Verification items for the finished model (mm, model axes). A direction names the side the tool comes from. Coordinates: 2 decimals unless noted, no trailing zeros. Order: outer loops, then holes, each group sorted by start corner. A loop starts at its lowest first (then second) coordinate and runs counter-clockwise, first axis right, second up. Notation, with made-up numbers: (-29.5, 71.5) - (-6.5, 71.5) arc R11 cw to (-6.5, 86.5) - close; hole circle Ø8 at (-15.75, 44.5). An arc over 180 degrees is marked (long way). Answer as CSV lines item,"result". Start each with the question number.
1. Set-up check for faces 5 (the flat face through (-100, -26, -142)), 6 (the flat face through (7.3, -15.1, -605)), 7 (the cylindrical face through (-15.738, -4.956, 3.479)), 8 (the flat face through (-100, -3, 18)), 9 (the cylindrical face through (124.307, -4.506, -623.07)): record each of +Z, -Z, +X, -X, +Y, -Y from which the full face is reachable in a straight line by a thin tool's end or side.
2. Section check A-A (z = -550). Record the cut outline in (x, y), and give its area (3 significant figures).
3. Material ranges on L1, parallel to Y at x = 0, z = -602.65; L2, parallel to Y at x = 0, z = -601; L3, parallel to X at y = 6.5, z = -95.5, recorded low to high. Write a range as [from, to].
4. Section check B-B (y = -63). Record the cut outline in (x, z).
5. Go/stop test with flat-tipped pins: pin 1 (5 mm diameter, centred on x = 73, z = -541.5, fed in from +Y); pin 2 (3.5 mm diameter, centred on x = 0, y = -25, fed in from +Z); pin 3 (2 mm diameter, centred on x = -24, y = -1, fed in from -Z). Record where each tip stops, or that it passes through.
6. Section check D-D (x = 110). Record the cut outline in (y, z).
7. Mould release check, pull along Z, two halves, no side actions. Record for faces 1 (the cylindrical face through (-95.693, 4.506, 22.93)), 2 (the cylindrical face through (120, 0, -609)), 3 (the cylindrical face through (-4.56, -34.7, -550.38)), 4 (the flat face through (0, 0, 2)): pulls with the +Z half, pulls with the -Z half, needs draft (parallel to the pull), parting line crosses it, or undercut.
from build123d import *

# Parameters (mm, degrees)
SKETCH3_W            = 300
SKETCH3_H            = 200
BOSS_EXTRUDE2_DEPTH  = 300
SKETCH8_R            = 35
SKETCH8_R_2          = 2
SKETCH8_R_3          = 2.3
BOSS_EXTRUDE7_DEPTH  = 5
BOSS_EXTRUDE8_DEPTH  = 300
SKETCH19_W           = 200
SKETCH19_H           = 260
CUT_EXTRUDE5_DEPTH   = 150
CUT_EXTRUDE3_REACH   = 673.584
CUT_EXTRUDE4_DEPTH   = 200
CHAMFER2_SIZE        = 50
SKETCH4_R            = 10
BOSS_EXTRUDE9_DEPTH  = 18
SKETCH15_R           = 15
BOSS_EXTRUDE10_DEPTH = 10
BOSS_EXTRUDE11_START = 18
SKETCH16_R           = 10
BOSS_EXTRUDE11_DEPTH = 18
BOSS_EXTRUDE12_START = 10
SKETCH17_R           = 15
BOSS_EXTRUDE12_DEPTH = 10
SKETCH18_R           = 75
BOSS_EXTRUDE13_DEPTH = 10
CUT_EXTRUDE6_REACH   = 685.318
SKETCH20_R           = 35
SKETCH21_R           = 16.5
CUT_EXTRUDE7_DEPTH   = 3
CUT_EXTRUDE8_START   = -3
SKETCH22_R           = 16.5
CUT_EXTRUDE8_DEPTH   = 3
SKETCH23_R           = 2
SKETCH23_R_2         = 2.3
CUT_EXTRUDE9_DEPTH   = 20


with BuildPart() as part:
    # Sketch3 → Boss-Extrude2 (new body)
    with BuildSketch(Plane.XY):
        Rectangle(SKETCH3_W, SKETCH3_H)
    extrude(amount=-BOSS_EXTRUDE2_DEPTH)

    # Sketch8 → Boss-Extrude7 (add)
    with BuildSketch(Plane.XY):
        Circle(SKETCH8_R)
        with Locations((0, 25)):
            Circle(SKETCH8_R_2, mode=Mode.SUBTRACT)
        with Locations((0, -25)):
            Circle(SKETCH8_R_2, mode=Mode.SUBTRACT)
        with Locations((25, 0)):
            Circle(SKETCH8_R_3, mode=Mode.SUBTRACT)
        with Locations((-25, 0)):
            Circle(SKETCH8_R_2, mode=Mode.SUBTRACT)
    extrude(amount=BOSS_EXTRUDE7_DEPTH)

    # Mirror1: part across plane


with BuildPart() as part_1:
    add(part.part)
    add(part.part.mirror(Plane(origin=(0, 0, -300), x_dir=(1, 0, 0), z_dir=(0, 0, -1))))

    # Sketch10 → Boss-Extrude8 (add)
    with BuildSketch(Plane(origin=(150, 0, 0), x_dir=(0, 0, -1), z_dir=(1, 0, 0))):
        Polygon((0, 100), (400, 250), (600, 100), align=None)
    extrude(amount=-BOSS_EXTRUDE8_DEPTH)

    # Sketch19 → Cut-Extrude5 (cut)
    with BuildSketch(Plane.XZ.offset(100)):
        with Locations((0, -140)):
            Rectangle(SKETCH19_W, SKETCH19_H)
    extrude(amount=-CUT_EXTRUDE5_DEPTH, mode=Mode.SUBTRACT)

    # Cut-Extrude3: up to this plane
    cut_extrude3_end = Plane(origin=(-768.465843843, 250, -400), z_dir=(0, 0.7999999999999999, -0.6000000000000001))
    # Sketch11 → Cut-Extrude3 (cut, up to the surface)
    with BuildSketch(Plane.XY, mode=Mode.PRIVATE) as cut_extrude3_sk1:
        Polygon((150, 100), (95.40446486, 250), (150, 250), align=None)
    cut_extrude3_tool1 = split(extrude(cut_extrude3_sk1.sketch, amount=-CUT_EXTRUDE3_REACH, mode=Mode.PRIVATE), bisect_by=cut_extrude3_end, keep=Keep.BOTH, mode=Mode.PRIVATE)
    add(cut_extrude3_tool1.solids().sort_by_distance((131.801488, 200, 0))[0], mode=Mode.SUBTRACT)
    # Sketch11 → Cut-Extrude3 (cut, up to the surface)
    with BuildSketch(Plane.XY, mode=Mode.PRIVATE) as cut_extrude3_sk2:
        Polygon((-150, 100), (-95.40446486, 250), (-150, 250), align=None)
    cut_extrude3_tool2 = split(extrude(cut_extrude3_sk2.sketch, amount=-CUT_EXTRUDE3_REACH, mode=Mode.PRIVATE), bisect_by=cut_extrude3_end, keep=Keep.BOTH, mode=Mode.PRIVATE)
    add(cut_extrude3_tool2.solids().sort_by_distance((-131.801488, 200, 0))[0], mode=Mode.SUBTRACT)

    # Sketch14 → Cut-Extrude4 (cut)
    with BuildSketch(Plane(origin=(0, 352, -264), x_dir=(1, 0, 0), z_dir=(0, 0.7999999999999999, -0.6000000000000002))):
        Polygon((-137.580501971, 410), (137.580501971, 410), (87.352609643, 180), (-87.352609643, 180), align=None)
    extrude(amount=-CUT_EXTRUDE4_DEPTH, mode=Mode.SUBTRACT)

    # Chamfer2
    chamfer2_edges = [part_1.edges().sort_by_distance(p)[0] for p in [
        (150, -100, -300),
        (-150, -100, -300),
    ]]
    chamfer(chamfer2_edges, length=CHAMFER2_SIZE - 0.0001)  # a hair under: the kernel refuses the full size

    # Sketch4 → Boss-Extrude9 (add)
    with BuildSketch(Plane.XY):
        with Locations(Location((-110, 0, 0), (0, 0, 180))):
            Circle(SKETCH4_R)
        with Locations(Location((110, 0, 0), (0, 0, 180))):
            Circle(SKETCH4_R)
    extrude(amount=BOSS_EXTRUDE9_DEPTH)

    # Sketch15 → Boss-Extrude10 (add)
    with BuildSketch(Plane.XY.offset(18)):
        with Locations((-110, 0)):
            Circle(SKETCH15_R)
        with Locations((110, 0)):
            Circle(SKETCH15_R)
    extrude(amount=BOSS_EXTRUDE10_DEPTH)

    # Sketch16 → Boss-Extrude11 (add)
    with BuildSketch(Plane(origin=(0, 0, -600), x_dir=(-1, 0, 0), z_dir=(0, 0, -1)).offset(BOSS_EXTRUDE11_START)):
        with Locations((110, 0)):
            Circle(SKETCH16_R)
        with Locations((-110, 0)):
            Circle(SKETCH16_R)
    extrude(amount=-BOSS_EXTRUDE11_DEPTH)

    # Sketch17 → Boss-Extrude12 (add)
    with BuildSketch(Plane(origin=(0, 0, -618), x_dir=(-1, 0, 0), z_dir=(0, 0, -1)).offset(BOSS_EXTRUDE12_START)):
        with Locations(Location((-110, 0, 0), (0, 0, 180))):
            Circle(SKETCH17_R)
        with Locations(Location((110, 0, 0), (0, 0, 180))):
            Circle(SKETCH17_R)
    extrude(amount=-BOSS_EXTRUDE12_DEPTH)

    # Sketch18 → Boss-Extrude13 (add)
    with BuildSketch(Plane(origin=(0, 87.671232877, 32.876712329), x_dir=(1, 0, 0), z_dir=(0, 0.9363291775690445, 0.35112344158839187))):
        with Locations(Location((0, 135.112344159, 0), (0, 0, 270))):
            Circle(SKETCH18_R)
    extrude(amount=BOSS_EXTRUDE13_DEPTH)

    # Cut-Extrude6: up to this plane
    cut_extrude6_end = Plane(origin=(-137.580501971, -54, -472), z_dir=(0, -0.6000000000000002, -0.7999999999999999))
    # Sketch20 → Cut-Extrude6 (cut, up to the surface)
    with BuildSketch(Plane(origin=(0, 0, -590), x_dir=(-1, 0, 0), z_dir=(0, 0, -1)), mode=Mode.PRIVATE) as cut_extrude6_sk1:
        with Locations(Location((0, 0, 0), (0, 0, 180))):
            Circle(SKETCH20_R)
    cut_extrude6_tool1 = split(extrude(cut_extrude6_sk1.sketch, amount=-CUT_EXTRUDE6_REACH, mode=Mode.PRIVATE), bisect_by=cut_extrude6_end, keep=Keep.BOTH, mode=Mode.PRIVATE)
    add(cut_extrude6_tool1.solids().sort_by_distance((0, 0, -590))[0], mode=Mode.SUBTRACT)

    # Sketch21 → Cut-Extrude7 (cut)
    with BuildSketch(Plane(origin=(0, 0, -605), x_dir=(-1, 0, 0), z_dir=(0, 0, -1))):
        Circle(SKETCH21_R)
    extrude(amount=-CUT_EXTRUDE7_DEPTH, mode=Mode.SUBTRACT)

    # Sketch22 → Cut-Extrude8 (cut)
    with BuildSketch(Plane.XY.offset(5).offset(CUT_EXTRUDE8_START)):
        with Locations(Location((0, 0, 0), (0, 0, 180))):
            Circle(SKETCH22_R)
    extrude(amount=CUT_EXTRUDE8_DEPTH, mode=Mode.SUBTRACT)

    # Sketch23 → Cut-Extrude9 (cut)
    with BuildSketch(Plane.XY.offset(5)):
        with Locations((0, 25)):
            Circle(SKETCH23_R)
        with Locations((25, 0)):
            Circle(SKETCH23_R_2)
        with Locations((0, -25)):
            Circle(SKETCH23_R)
        with Locations((-25, 0)):
            Circle(SKETCH23_R)
    extrude(amount=-CUT_EXTRUDE9_DEPTH, mode=Mode.SUBTRACT)


solid = part_1.part
Evaluation:
1,face 5,"-Y"
1,face 6,"-Z, +Y, -Y"
1,face 7,"+Z"
1,face 8,"none"
1,face 9,"-Z"
2,outline,"(-150, -50) - (-100, -100) - (100, -100) - (150, -50) - (150, 100) - (136.35, 137.5) - (126.12, 137.5) - (137.58, 50) - (-137.58, 50) - (-126.12, 137.5) - (-136.35, 137.5) - (-150, 100) - close; hole circle Ø70 at (0, 0)"
2,area,"41,300 mm²"
3,L1,"y = [-35, -27], [-23, -16.5], [16.5, 23], [27, 35]"
3,L2,"y = [-35, -27], [-23, 23], [27, 35]"
3,L3,"x = [-150, -100], [100, 150]"
4,outline,"(-137, -600) - (137, -600) - (137, 0) - (-137, 0) - close; hole (-100, -270) - (100, -270) - (100, -10) - (-100, -10) - close"
5,pin 1,"stops at y = 42"
5,pin 2,"stops at z = -270"
5,pin 3,"stops at z = -605"
6,outline,"(-90, -600) - (-10, -600) - (-10, -618) - (-15, -618) - (-15, -628) - (15, -628) - (15, -618) - (10, -618) - (10, -600) - (100, -600) - (106, -592) - (-54, -472) - (21.78, -370.96) - (181.78, -490.96) - (209.9, -453.47) - (209.9, -293.06) - (100, 0) - (10, 0) - (10, 18) - (15, 18) - (15, 28) - (-15, 28) - (-15, 18) - (-10, 18) - (-10, 0) - (-90, 0) - close"
7,face 1,"needs draft"
7,face 2,"undercut"
7,face 3,"undercut"
7,face 4,"pulls with the +Z half"
